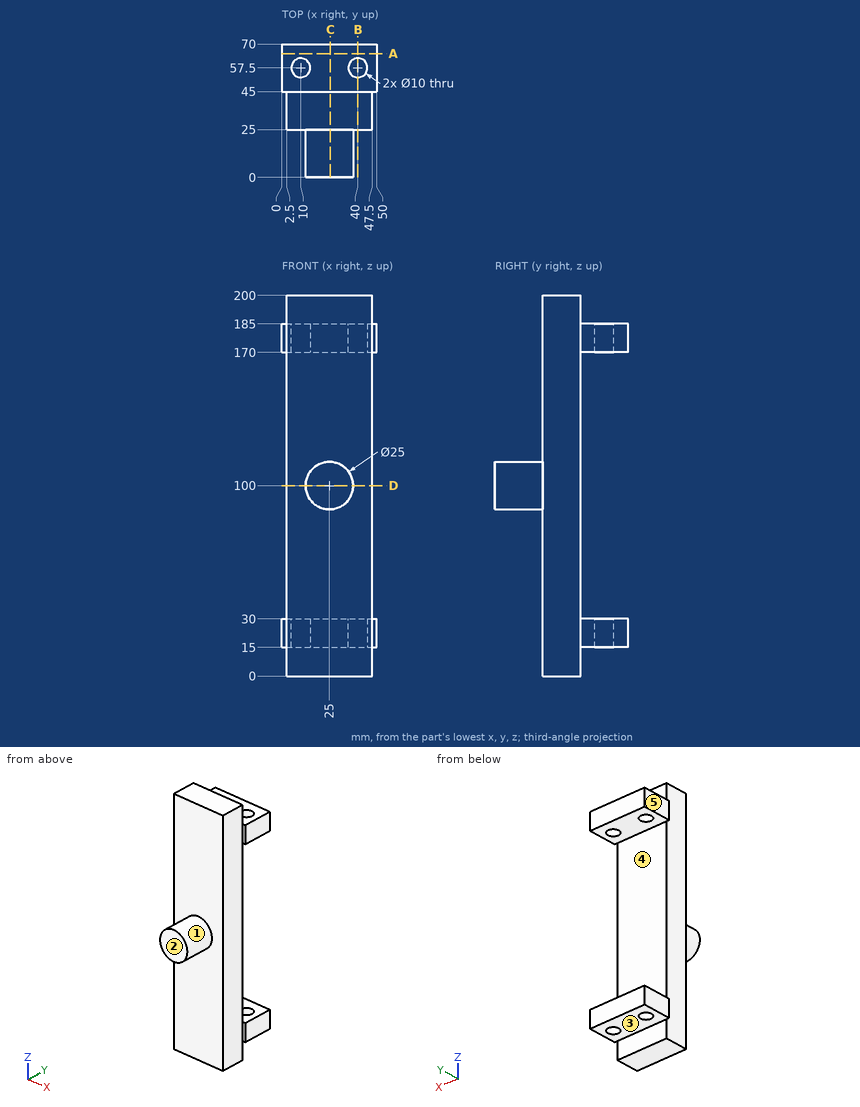
For this review, use the dimensioned drawing (mm, ordinates from the lowest corner) and the shaded views. A direction names the side the tool comes from. Give positions to 0.01 mm unless a question says otherwise; leave off trailing zeros. Loops run counter-clockwise (first coordinate to the right, second up) from the corner with the lowest first, then second, coordinate; pieces in that order, holes last. Notation, with made-up numbers: (20, 79.5) -> (27, 79.5) arc R10 cw to (27, 90.5) -> close; hole circle Ø10 at (14.5, -13.5). An arc over 180 degrees is marked (long way). One line per question, with ' | ' between items. Start each with the question number.
(1) For the marked faces 1, 2, 3, 4 and 5, list the 3-axis set-ups (+Z, -Z, +X, -X, +Y, -Y) from which the entire face can be reached by the end or side of a thin tool; tool diameter is ignored.
(2) For line 1 (X direction, y = 57, z = 26); line 2 (Y direction, x = 10, z = 173); line 3 (Z direction, x = 29, y = 61.5), list the stretches that pass through material, from the lowest coordinate up.
(3) We need section B-B (x = 40). State the section outline as (y, z) points, and give its area (3 significant figures).
(4) We need section D-D (z = 100). State the section outline as (x, y) points.
(5) Insertion check: P1, Ø12.5, axis at x = 21, y = 59.5, coming from the +Z side; P2, Ø4, axis at x = 38.5, z = 117, coming from the -Y side; P3, Ø4.5, axis at x = 15.5, z = 192.5, coming from the +Y side; P4, Ø13.5, axis at x = 23, z = 117, coming from the -Y side. Each pin has a flat end and moves straight along its axis. Give the tip position at first contact, or say it passes through.
(6) We need section A-A (y = 65). State the section outline as (x, z) points, and give its area (3 significant figures).
(7) We need section C-C (x = 25.5). State the section outline as (y, z) points.
The answers:
1) face 1: -Y | face 2: +Z, -Z, +X, -X, -Y | face 3: -Z, +X, -X, +Y | face 4: +X, -X, +Y | face 5: +Z, -Z, -X, +Y, -Y
2) line 1: x = 0 to 5.03, 14.97 to 35.03, 44.97 to 50 | line 2: y = 25 to 52.5, 62.5 to 70 | line 3: z = 15 to 30, 170 to 185
3) outline: (25, 0) -> (45, 0) -> (45, 15) -> (52.5, 15) -> (52.5, 30) -> (45, 30) -> (45, 170) -> (52.5, 170) -> (52.5, 185) -> (45, 185) -> (45, 200) -> (25, 200) -> close; (62.5, 15) -> (70, 15) -> (70, 30) -> (62.5, 30) -> close; (62.5, 170) -> (70, 170) -> (70, 185) -> (62.5, 185) -> close | area: 4,450 mm^2
4) outline: (2.5, 25) -> (12.5, 25) -> (12.5, 0) -> (37.5, 0) -> (37.5, 25) -> (47.5, 25) -> (47.5, 45) -> (2.5, 45) -> close
5) P1: stops at z = 185 | P2: stops at y = 25 | P3: stops at y = 45 | P4: stops at y = 0
6) outline: (0, 15) -> (50, 15) -> (50, 30) -> (0, 30) -> close; (0, 170) -> (50, 170) -> (50, 185) -> (0, 185) -> close | area: 1,500 mm^2
7) outline: (0, 87.51) -> (25, 87.51) -> (25, 0) -> (45, 0) -> (45, 15) -> (70, 15) -> (70, 30) -> (45, 30) -> (45, 170) -> (70, 170) -> (70, 185) -> (45, 185) -> (45, 200) -> (25, 200) -> (25, 112.49) -> (0, 112.49) -> close
